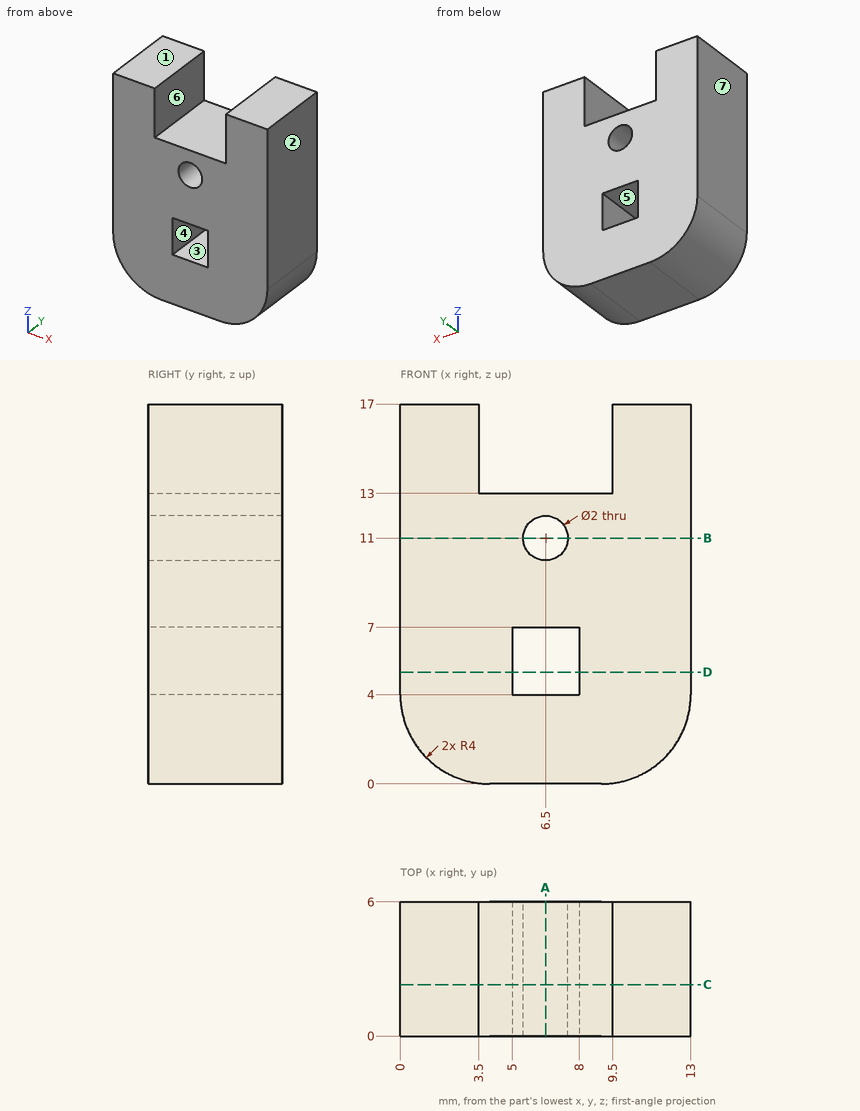
The figure shows three views and two pictorial views of one solid part (mm, origin at its lowest corner). Answer the questions. A direction names the side the tool comes from. Coordinates: 2 decimals unless noted, no trailing zeros. Loops run counter-clockwise (first coordinate to the right, second up) from the corner with the lowest first, then second, coordinate; pieces in that order, holes last.
(1) Consider line 1 along X through (y, z) = (1.7, 11); line 2 along X through (y, z) = (0.75, 6.75); line 3 along Z through (x, y) = (4, 5.3). Determine where each line is inside the solid, lowest interval first.
Solution:
line 1: x = 0 to 5.5, 7.5 to 13
line 2: x = 0 to 5, 8 to 13
line 3: z = 0 to 13
(2) A tool of negligible diameter and unlimited length cuts with its end or side. For the marked faces 5, 6 and 7, from which of +Z, -Z, +X, -X, +Y, -Y can it reach the whole face along a straight path? Write none if from no direction.
Solution:
face 5: +Y, -Y
face 6: +Z, +Y, -Y
face 7: +Z, -Z, -X, +Y, -Y
(3) Flat-ended cylindrical pins translate along their axes: pin 1 Ø3.5 at (x, y) = (6, 3.5) entering from -Z; pin 2 Ø1.5 at (x, y) = (6.5, 2.5) entering from +Z. Find the tip coordinate at first contact, or state that the pin passes through.
Solution:
pin 1: stops at z = 0
pin 2: stops at z = 13
(4) The mould has two halves that part along Z. Classify the marked faces 1, 2, 3 and 4: released by +Z, released by -Z, zero draft, split by the parting line, or undercut.
Solution:
face 1: released by +Z
face 2: zero draft
face 3: undercut
face 4: undercut
(5) The part is cut by section A-A (x = 6.5). Determine the outline of the cut face in (y, z).
Solution:
outline: (0, 0) - (6, 0) - (6, 4) - (0, 4) - close; (0, 7) - (6, 7) - (6, 10) - (0, 10) - close; (0, 12) - (6, 12) - (6, 13) - (0, 13) - close
(6) The part is cut by section C-C (y = 2.3). Determine the outline of the cut face in (x, z), and give its area (3 significant figures).
Solution:
outline: (0, 4) arc R4 ccw to (4, 0) - (9, 0) arc R4 ccw to (13, 4) - (13, 17) - (9.5, 17) - (9.5, 13) - (3.5, 13) - (3.5, 17) - (0, 17) - close; hole (5, 4) - (8, 4) - (8, 7) - (5, 7) - close; hole circle Ø2 at (6.5, 11)
area: 178 mm2
(7) The part is cut by section D-D (z = 5). Determine the outline of the cut face in (x, y).
Solution:
outline: (0, 0) - (5, 0) - (5, 6) - (0, 6) - close; (8, 0) - (13, 0) - (13, 6) - (8, 6) - close
(8) The part is cut by section B-B (z = 11). Determine the outline of the cut face in (x, y).
Solution:
outline: (0, 0) - (5.5, 0) - (5.5, 6) - (0, 6) - close; (7.5, 0) - (13, 0) - (13, 6) - (7.5, 6) - close
